```python
from build123d import *

# Parameters (mm, degrees)
BOSS_EXTRUDE1_DEPTH = 8.75
FILLET1_R           = 2
CHAMFER1_SIZE       = 3
CHAMFER1_SIZE2      = 1.732050808
FILLET2_R           = 3


with BuildPart() as part:
    # Sketch1 → Boss-Extrude1 (new, symmetric)
    with BuildSketch(Plane(origin=(0, 0, 0), x_dir=(1, 0, 0), z_dir=(0, 1, 0))):
        Polygon((0, 39.05), (0, -39.05), (-40, -39.05), (-40, -46.05), (9, -46.05), (9, 47.45), (-20.5, 47.45), (-20.5, 39.05), align=None)
    extrude(amount=BOSS_EXTRUDE1_DEPTH, both=True)

    # Fillet1
    fillet1_edges = [part.edges().sort_by_distance(p)[0] for p in [
        (9, 0, -47.45),
        (9, 0, 46.05),
    ]]
    fillet(fillet1_edges, radius=FILLET1_R)

    # Chamfer1
    chamfer1_edges = [part.edges().sort_by_distance(p)[0] for p in [
        (-20.5, 0, -47.45),
    ]]
    chamfer1_side = [part.faces().sort_by_distance(p)[0] for p in [
        (-6.75, 0, -47.45),
    ]]
    chamfer(chamfer1_edges, length=CHAMFER1_SIZE, length2=CHAMFER1_SIZE2, reference=chamfer1_side[0])

    # Fillet2
    fillet2_edges = [part.edges().sort_by_distance(p)[0] for p in [
        (-40, 0, 46.05),
    ]]
    fillet(fillet2_edges, radius=FILLET2_R)


solid = part.part
```
Geometry: final body of the model. Coordinates: model frame, mm. A direction names the side the tool comes from. Round coordinates to 2 decimals unless told otherwise and drop trailing zeros. Loops run counter-clockwise (first coordinate to the right, second up) from the corner with the lowest first, then second, coordinate; pieces in that order, holes last. Notation, with made-up numbers: (72, -22.5) -> (113, -22.5) arc R29 cw to (113, 6.5) -> close; hole circle Ø5 at (17, 56). An arc over 180 degrees is marked (long way). Use one line per item in the form item = value. Start each with the question number.
1) Access query for faces 1 (the flat face through (1, 8.75, 3)), 2 (the flat face through (-20.5, 0, -42)), 3 (the flat face through (0, 0, -1)). Directions: +Z, -Z, +X, -X, +Y, -Y. A direction counts if a zero-diameter tool reaches every point of the face in a straight line with its end or side. Return the directions, or none.
2) Section C-C on z = 5.5. Output: boundary loops of the cut face in (x, y), then the cut area to 4 significant figures.
3) Section B-B on y = -7.5. Output: boundary loops of the cut face in (x, z).
4) Draft query along Z for faces 4 (the flat face through (-10, 0, -39.05)), 5 (the flat face through (-40, 0, 41)), 6 (the flat face through (-19.021, 0.122, -46.572)). Return one class per face: released by +Z, released by -Z, zero draft, split by the parting line, or undercut.
5) First-contact query: P1, Ø3.5, axis at y = -4, z = -43, coming from the -X side; P2, Ø9, axis at y = 2.5, z = 3, coming from the -X side. Flat tips, straight axial feed; report the tip coordinate or a pass-through.
6) Section D-D on x = -36. Output: boundary loops of the cut face in (y, z).
7) Line query: L1, parallel to Z at x = -14, y = 0.75; L2, parallel to Z at x = -27, y = 7.75; L3, parallel to X at y = 0.5, z = 12.5. Output: solid intervals per line, ascending.
8) Section A-A on x = -15. Output: boundary loops of the cut face in (y, z), then the cut area to 4 significant figures.
Response:
q1.face_1 = +Z, -Z, +X, -X, +Y
q1.face_2 = -Z, -X, +Y, -Y
q1.face_3 = -X, +Y, -Y
q2.outline = (0, -8.75) -> (9, -8.75) -> (9, 8.75) -> (0, 8.75) -> close
q2.area = 157.5 mm^2
q3.outline = (-40, 39.05) -> (0, 39.05) -> (0, -39.05) -> (-20.5, -39.05) -> (-20.5, -45.72) -> (-17.5, -47.45) -> (7, -47.45) arc R2 ccw to (9, -45.45) -> (9, 44.05) arc R2 ccw to (7, 46.05) -> (-37, 46.05) arc R3 ccw to (-40, 43.05) -> close
q4.face_4 = undercut
q4.face_5 = zero draft
q4.face_6 = released by -Z
q5.P1 = -20.5
q5.P2 = 0
q6.outline = (-8.75, 39.05) -> (8.75, 39.05) -> (8.75, 46.05) -> (-8.75, 46.05) -> close
q7.L1 = -47.45 to -39.05, 39.05 to 46.05
q7.L2 = 39.05 to 46.05
q7.L3 = 0 to 9
q8.outline = (-8.75, -47.45) -> (8.75, -47.45) -> (8.75, -39.05) -> (-8.75, -39.05) -> close; (-8.75, 39.05) -> (8.75, 39.05) -> (8.75, 46.05) -> (-8.75, 46.05) -> close
q8.area = 269.5 mm^2
